CAD build for the part. Positions are in the model's coordinates, mm. A direction names the side the tool comes from. Give positions to 0.01 mm unless a question says otherwise; leave off trailing zeros. Loops run counter-clockwise (first coordinate to the right, second up) from the corner with the lowest first, then second, coordinate; pieces in that order, holes last. Notation, with made-up numbers: M 41.25,-27 L 79.25,-27 A35 ccw 79.25,5 Z; hole C 84,67 d11. An arc over 180 degrees is marked long. One line per question, with ' | ' between items.
```python
from build123d import *

# Parameters (mm, degrees)
BOSS_EXTRUDE1_DEPTH   = 6.35
SKETCH2_W             = 60.96
SKETCH2_H             = 49.53
CUT_EXTRUDE1_DEPTH    = 0.635
SKETCH5_W             = 7.874
SKETCH5_H             = 5.334
BOSS_EXTRUDE2_DEPTH   = 31.75
BOSS_EXTRUDE2_2_DEPTH = 31.75
SKETCH7_R             = 1.55575
CUT_EXTRUDE2_DEPTH    = 169.168334118
BOSS_EXTRUDE3_START   = -8.255
BOSS_EXTRUDE3_DEPTH   = 34.29
SKETCH9_R             = 1.7399
SKETCH9_W             = 24.13
SKETCH9_H             = 16.891
CUT_EXTRUDE3_DEPTH    = 175.333671147
SKETCH11_W            = 18.796
SKETCH11_H            = 70.745386066
BOSS_EXTRUDE6_DEPTH   = 6.35
FILLET1_R             = 8.255


with BuildPart() as part:
    # Sketch1 → Boss-Extrude1 (new body)
    with BuildSketch(Plane(origin=(0, 0, 0), x_dir=(1, 0, 0), z_dir=(0, 1, 0))):
        Polygon((-25.4, 38.1), (-61.595, 38.1), (-61.595, -38.1), (61.595, -38.1), (61.595, 38.1), (25.4, 38.1), (25.4, 107.95), (-25.4, 107.95), align=None)
    extrude(amount=BOSS_EXTRUDE1_DEPTH)

    # Sketch2 → Cut-Extrude1 (cut)
    with BuildSketch(Plane(origin=(0, 6.35, 0), x_dir=(1, 0, 0), z_dir=(0, 1, 0))):
        Rectangle(SKETCH2_W, SKETCH2_H)
    extrude(amount=-CUT_EXTRUDE1_DEPTH, mode=Mode.SUBTRACT)


with BuildPart() as body_2:
    # Sketch5 → Boss-Extrude2 (new body)
    with BuildSketch(Plane(origin=(0, 6.35, 0), x_dir=(1, 0, 0), z_dir=(0, 1, 0))):
        with Locations((-46.736, -35.312386066)):
            Rectangle(SKETCH5_W, SKETCH5_H)
    boss_extrude2 = extrude(amount=BOSS_EXTRUDE2_DEPTH)


with BuildPart() as body_3:
    # Sketch5 → Boss-Extrude2 2 (new body)
    with BuildSketch(Plane(origin=(0, 6.35, 0), x_dir=(1, 0, 0), z_dir=(0, 1, 0))):
        with Locations((-57.658, -35.312386066)):
            Rectangle(SKETCH5_W, SKETCH5_H)
    boss_extrude2_2 = extrude(amount=BOSS_EXTRUDE2_2_DEPTH)


with BuildPart() as part_1:
    add(part.part)

    # Mirror4: Boss-Extrude2, Boss-Extrude2 2 across plane
    add(boss_extrude2.mirror(Plane(origin=(0, 0, 0), x_dir=(0, 0, 1), z_dir=(1, 0, 0))))
    add(boss_extrude2_2.mirror(Plane(origin=(0, 0, 0), x_dir=(0, 0, 1), z_dir=(1, 0, 0))))


with BuildPart() as cut_extrude2_tool:
    # Sketch7 → Cut-Extrude2 (new, through all)
    with BuildSketch(Plane(origin=(61.595, 0, 0), x_dir=(0, 0, -1), z_dir=(1, 0, 0))):
        with Locations((-35.312386066, 25.4)):
            Circle(SKETCH7_R)
    extrude(amount=-CUT_EXTRUDE2_DEPTH)


with BuildPart() as part_2:
    add(part_1.part)

    # Cut-Extrude2: cut by cut_extrude2_tool
    add(cut_extrude2_tool.part, mode=Mode.SUBTRACT)

    # Sketch8 → Boss-Extrude3 (add)
    with BuildSketch(Plane(origin=(25.4, 0, 0), x_dir=(0, 0, -1), z_dir=(1, 0, 0)).offset(BOSS_EXTRUDE3_START)):
        Polygon((111.616174209, 0), (149.716174209, 65.991135768), (144.216912895, 69.166135768), (107.95, 6.35), (107.95, 0), align=None)
    extrude(amount=-BOSS_EXTRUDE3_DEPTH)

    # Sketch9 → Cut-Extrude3 (cut, through all)
    with BuildSketch(Plane(origin=(0, -45.156221169, -78.212869343), x_dir=(1, 0, 0), z_dir=(0, 0.49999999999997874, 0.866025403784451))):
        with Locations(Location((-14.2113, 129.074387105, 0), (0, 0, 270))):
            Circle(SKETCH9_R)
        with Locations(Location((14.2113, 129.074387105, 0), (0, 0, 90))):
            Circle(SKETCH9_R)
        with Locations(Location((14.2113, 100.651787105, 0), (0, 0, 270))):
            Circle(SKETCH9_R)
        with Locations(Location((-14.2113, 100.651787105, 0), (0, 0, 90))):
            Circle(SKETCH9_R)
        with Locations((0, 118.868787105)):
            Rectangle(SKETCH9_W, SKETCH9_H)
    extrude(amount=-CUT_EXTRUDE3_DEPTH, mode=Mode.SUBTRACT)



with BuildPart() as body_2_1:
    add(body_2.part)

    # Cut-Extrude2: cut by cut_extrude2_tool
    add(cut_extrude2_tool.part, mode=Mode.SUBTRACT)


with BuildPart() as body_3_1:
    add(body_3.part)

    # Cut-Extrude2: cut by cut_extrude2_tool
    add(cut_extrude2_tool.part, mode=Mode.SUBTRACT)


with BuildPart() as part_3:
    add(part_2.part)

    add(body_2_1.part)  # Boss-Extrude6 merges body 2

    add(body_3_1.part)  # Boss-Extrude6 merges body 3
    # Sketch11 → Boss-Extrude6 (add)
    with BuildSketch(Plane(origin=(0, 6.35, 0), x_dir=(1, 0, 0), z_dir=(0, 1, 0))):
        with Locations((-52.197, 2.727306967)):
            Rectangle(SKETCH11_W, SKETCH11_H)
        with Locations((52.197, 2.727306967)):
            Rectangle(SKETCH11_W, SKETCH11_H)
    extrude(amount=BOSS_EXTRUDE6_DEPTH)

    # Fillet1
    # the kernel refuses this fillet: 8.255 mm, written as the material it adds along each edge
    with BuildSketch(Plane(origin=(-17.145, 26.9875, -107.95), x_dir=(-1, 0, 0), z_dir=(0, -1, 0))) as fillet1_piece_1_section:
        with BuildLine():
            CenterArc((FILLET1_R, FILLET1_R), FILLET1_R, 180, 90)
            Line((0, FILLET1_R), (0, 0))
            Line((0, 0), (FILLET1_R, 0))
        make_face()
    fillet1_piece_1 = extrude(amount=26.9875, mode=Mode.PRIVATE)
    fillet1_piece_1 = split(fillet1_piece_1, bisect_by=Plane(origin=(-18.026106342, 6.35, -111.490654818), z_dir=(0, 1, 0)), keep=Keep.TOP, mode=Mode.PRIVATE)
    fillet1_piece_1 = split(fillet1_piece_1, bisect_by=Plane(origin=(-18.026106342, 10.193700171, -110.169161328), z_dir=(0, -0.4999999999999879, -0.8660254037844457)), keep=Keep.TOP, mode=Mode.PRIVATE)
    fillet1_piece_1 = split(fillet1_piece_1, bisect_by=Plane(origin=(-18.026106342, 7.018700171, -115.668422642), z_dir=(0, 0.49999999999999845, 0.8660254037844396)), keep=Keep.TOP, mode=Mode.PRIVATE)
    add(fillet1_piece_1)
    with BuildSketch(Plane(origin=(-17.145, 6.35, -107.95), x_dir=(-1, 0, 0), z_dir=(0, -1, 0))) as fillet1_piece_2_section:
        with BuildLine():
            CenterArc((FILLET1_R, FILLET1_R), FILLET1_R, 180, 90)
            Line((0, FILLET1_R), (0, 0))
            Line((0, 0), (FILLET1_R, 0))
        make_face()
    fillet1_piece_2 = extrude(amount=6.35, mode=Mode.PRIVATE)
    fillet1_piece_2 = split(fillet1_piece_2, bisect_by=Plane(origin=(-19.126244344, 4.717934574, -107.007726587), z_dir=(0, -0.4999999999999879, -0.8660254037844457)), keep=Keep.TOP, mode=Mode.PRIVATE)
    fillet1_piece_2 = split(fillet1_piece_2, bisect_by=Plane(origin=(-19.126244344, 1.542934574, -112.506987901), z_dir=(0, 0.49999999999999845, 0.8660254037844396)), keep=Keep.TOP, mode=Mode.PRIVATE)
    add(fillet1_piece_2)
    with BuildSketch(Plane(origin=(17.145, 26.9875, -107.95), x_dir=(1, 0, 0), z_dir=(0, -1, 0))) as fillet1_piece_3_section:
        with BuildLine():
            CenterArc((FILLET1_R, -FILLET1_R), FILLET1_R, 90, 90)
            Line((0, -FILLET1_R), (0, 0))
            Line((0, 0), (FILLET1_R, 0))
        make_face()
    fillet1_piece_3 = extrude(amount=26.9875, mode=Mode.PRIVATE)
    fillet1_piece_3 = split(fillet1_piece_3, bisect_by=Plane(origin=(18.026106342, 6.35, -111.490654818), z_dir=(0, 1, 0)), keep=Keep.TOP, mode=Mode.PRIVATE)
    fillet1_piece_3 = split(fillet1_piece_3, bisect_by=Plane(origin=(18.026106342, 10.193700171, -110.169161328), z_dir=(0, -0.4999999999999879, -0.8660254037844457)), keep=Keep.TOP, mode=Mode.PRIVATE)
    fillet1_piece_3 = split(fillet1_piece_3, bisect_by=Plane(origin=(18.026106342, 7.018700171, -115.668422642), z_dir=(0, 0.49999999999999845, 0.8660254037844396)), keep=Keep.TOP, mode=Mode.PRIVATE)
    add(fillet1_piece_3)
    with BuildSketch(Plane(origin=(17.145, 6.35, -107.95), x_dir=(1, 0, 0), z_dir=(0, -1, 0))) as fillet1_piece_4_section:
        with BuildLine():
            CenterArc((FILLET1_R, -FILLET1_R), FILLET1_R, 90, 90)
            Line((0, -FILLET1_R), (0, 0))
            Line((0, 0), (FILLET1_R, 0))
        make_face()
    fillet1_piece_4 = extrude(amount=6.35, mode=Mode.PRIVATE)
    fillet1_piece_4 = split(fillet1_piece_4, bisect_by=Plane(origin=(19.126244344, 4.717934574, -107.007726587), z_dir=(0, -0.4999999999999879, -0.8660254037844457)), keep=Keep.TOP, mode=Mode.PRIVATE)
    fillet1_piece_4 = split(fillet1_piece_4, bisect_by=Plane(origin=(19.126244344, 1.542934574, -112.506987901), z_dir=(0, 0.49999999999999845, 0.8660254037844396)), keep=Keep.TOP, mode=Mode.PRIVATE)
    add(fillet1_piece_4)
    with BuildSketch(Plane(origin=(-25.4, 0, -38.1), x_dir=(-1, 0, 0), z_dir=(0, 1, 0)), Plane(origin=(25.4, 0, -38.1), x_dir=(0, 0, -1), z_dir=(0, 1, 0))) as fillet1_piece_5:
        with BuildLine():
            CenterArc((FILLET1_R, -FILLET1_R), FILLET1_R, 90, 90)
            Line((0, -FILLET1_R), (0, 0))
            Line((0, 0), (FILLET1_R, 0))
        make_face()
    extrude(amount=6.35)


solid = part_3.part
```
Item 1: Drop flat-ended pins along their axis: P1, Ø4, axis at x = 45.5, y = 27.5, coming from the +Z side; P2, Ø6, axis at x = 2, y = 11.5, coming from the -Z side; P3, Ø6, axis at x = -46, z = 34.5, coming from the +Y side; P4, Ø1.9, axis at y = 25.4, z = 35.31, coming from the +X side. Give the stop position or say it passes through.
Conclusion:
P1: z = 37.98 | P2: z = -119.99 | P3: y = 38.1 | P4: through
Item 2: Saw through at B-B on y = 18.5. Give the cut face in (x, z) (3 decimals).
Conclusion:
outline: M -61.595,32.645 L -53.721,32.645 L -53.721,37.979 L -61.595,37.979 Z; M -50.673,32.645 L -42.799,32.645 L -42.799,37.979 L -50.673,37.979 Z; M -17.239,-114.965 A8.255 cw -17.145,-116.205 L -17.145,-122.297 L 17.145,-122.297 L 17.145,-116.205 A8.255 cw 17.239,-114.965 Z; M 42.799,32.645 L 50.673,32.645 L 50.673,37.979 L 42.799,37.979 Z; M 53.721,32.645 L 61.595,32.645 L 61.595,37.979 L 53.721,37.979 Z
Item 3: Saw through at C-C on x = -48.5. Give the cut face in (y, z), and give its area (3 significant figures).
Conclusion:
outline: M 0,-38.1 L 12.7,-38.1 L 12.7,32.65 L 38.1,32.65 L 38.1,37.98 L 6.35,37.98 L 6.35,38.1 L 0,38.1 Z; hole C 25.4,35.31 d3.11 | area: 1,090 mm²
Item 4: Drill centre lines: line 1 along X through (y, z) = (7.5, -0.5) (3 decimals); line 2 along Z through (x, y) = (-45, 23); line 3 along Y through (x, z) = (24, -70). Where is each one in solid material? Low to high. Write a range as [from, to].
Conclusion:
line 1: [-61.595, -42.799], [42.799, 61.595] | line 2: [32.65, 37.98] | line 3: [0, 6.35]
Item 5: Mould opens along Z. For faces 4 (the flat face through (42.799, 12, 9)), 5 (the cylindrical face through (-15.755, 64.365, -145.06)), 6 (the flat face through (47, 22, 37.979)) say: pulls with the +Z half, pulls with the -Z half, needs draft (parallel to the pull), parting line crosses it, or undercut.
Conclusion:
face 4: needs draft | face 5: undercut | face 6: pulls with the +Z half
Item 6: Saw through at A-A on x = -1.5. Give the cut face in (y, z) (3 decimals), and give its area (3 significant figures).
Conclusion:
outline: M 0,-111.616 L 47.298,-138.924 L 50.473,-133.425 L 6.35,-107.95 L 6.35,-24.765 L 5.715,-24.765 L 5.715,24.765 L 6.35,24.765 L 6.35,38.1 L 0,38.1 Z; M 61.926,-147.369 L 65.991,-149.716 L 69.166,-144.217 L 65.101,-141.87 Z | area: 1,270 mm²
Item 7: Saw through at D-D on z = 18. Give the cut face in (x, y) (3 decimals).
Conclusion:
outline: M -61.595,0 L 61.595,0 L 61.595,12.7 L 42.799,12.7 L 42.799,6.35 L 30.48,6.35 L 30.48,5.715 L -30.48,5.715 L -30.48,6.35 L -42.799,6.35 L -42.799,12.7 L -61.595,12.7 Z
Item 8: 3-axis set-ups, long thin cutter, end or side, ignore diameter. For faces 1 (the flat face through (0, 5.715, 0)), 2 (the flat face through (47, 25, 32.645)), 3 (the flat face through (-50.673, 22, 35)): which of +Z, -Z, +X, -X, +Y, -Y reach the whole face in a straight line?
Conclusion:
face 1: +Y | face 2: -Z, +X, -X, +Y | face 3: +Z, +Y
